Geometry check sheet. Reference: drawing and pictorial views, mm from the part's lowest x, y, z. A direction names the side the tool comes from. Coordinates: 2 decimals unless noted, no trailing zeros. Write each loop counter-clockwise with the first axis right and the second up, starting at its lowest first coordinate (ties: lowest second). Pieces come first, ordered by that corner, then holes. Notation, with made-up numbers: (-6.5, 2.25) - (50.5, 2.25) arc R23 cw to (50.5, 37.25) - close; hole circle Ø6 at (16, 42.25). An arc over 180 degrees is marked (long way). Use one line per item in the form item = value. Start each with the question number.
(1) Tool access check on the marked faces 4, 5, 6, 7 and 8. Record the directions out of +Z, -Z, +X, -X, +Y, -Y that give a thin tool (end or side, any length) a straight path to the whole face; none if there is none.
(2) Gauge pin test, flat ends, axial feed: pin 1 Ø4 at (x, z) = (9, 8) entering from +Y; pin 2 Ø2 at (y, z) = (24.5, 18) entering from -X; pin 3 Ø1.5 at (x, z) = (11, 17.5) entering from -Y; pin 4 Ø4 at (x, y) = (10, 23.5) entering from -Z. Record the tip position at first contact, or that the pin passes through.
(3) Sectioned sample at C-C (y = 2.75). Record the cut outline in (x, z).
(4) Sectioned sample at B-B (z = 14.5). Record the cut outline in (x, y).
(5) Sectioned sample at A-A (x = 10). Record the cut outline in (y, z) (1 decimal).
(6) Sectioned sample at D-D (z = 3). Record the cut outline in (x, y) (1 decimal), and give its area (3 significant figures).
(7) Mould release check, pull along Z, two halves, no side actions. Record for the marked faces 1, 2 and 3: released by +Z, released by -Z, zero draft, split by the parting line, or undercut.
(8) Material ranges on line 1 (Y direction, x = 10, z = 1.8) (1 decimal); line 2 (X direction, y = 8, z = 14); line 3 (Z direction, x = 6.25, y = 11), recorded low to high. Write a range as [from, to].
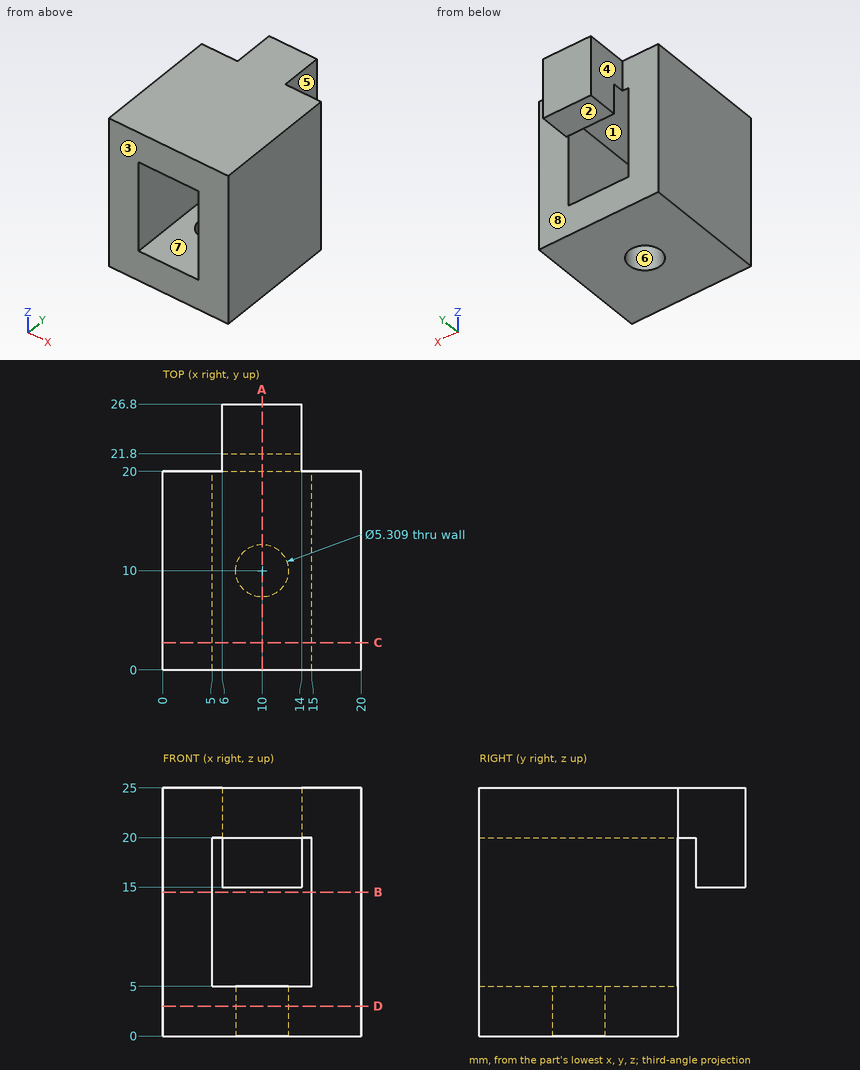
Answers below:
q1.face_4 = +Z, -Z, -X, +Y
q1.face_5 = +Z, -Z, +X, +Y
q1.face_6 = -Z
q1.face_7 = +Y, -Y
q1.face_8 = -Z, +Y
q2.pin_1 = through
q2.pin_2 = 6
q2.pin_3 = 21.8
q2.pin_4 = 15
q3.outline = (0, 0) - (20, 0) - (20, 25) - (0, 25) - close; hole (5, 5) - (15, 5) - (15, 20) - (5, 20) - close
q4.outline = (0, 0) - (5, 0) - (5, 20) - (0, 20) - close; (15, 0) - (20, 0) - (20, 20) - (15, 20) - close
q5.outline = (0, 0) - (7.3, 0) - (7.3, 5) - (0, 5) - close; (0, 20) - (21.8, 20) - (21.8, 15) - (26.8, 15) - (26.8, 25) - (0, 25) - close; (12.7, 0) - (20, 0) - (20, 5) - (12.7, 5) - close
q6.outline = (0, 0) - (20, 0) - (20, 20) - (0, 20) - close; hole circle Ø5.3 at (10, 10)
q6.area = 378 mm2
q7.face_1 = undercut
q7.face_2 = released by -Z
q7.face_3 = zero draft
q8.line_1 = [0, 7.3], [12.7, 20]
q8.line_2 = [0, 5], [15, 20]
q8.line_3 = [0, 5], [20, 25]
